Check sheet for the drawn part. Datum: minimum x, y, z corner. Units: mm. Round coordinates to 2 decimals unless told otherwise and drop trailing zeros. Write each loop counter-clockwise with the first axis right and the second up, starting at its lowest first coordinate (ties: lowest second). Pieces come first, ordered by that corner, then holes. Notation, with made-up numbers: (73, 25.5) - (124, 25.5) arc R22 ccw to (124, 52.5) - close; hole circle Ø11 at (-23, 5.5). An arc over 180 degrees is marked (long way). Answer as a JSON object with one key per item and string values. Group by question number.
Item 1: Gauge pin test, flat ends, axial feed: P1, Ø0.9, axis at y = 52, z = 2, coming from the +X side; P2, Ø1, axis at x = 209, z = 1, coming from the -Y side; P3, Ø1.5, axis at x = 117, z = 1, coming from the +Y side. Record the tip position at first contact, or that the pin passes through.
Item 2: Sectioned sample at B-B on x = 108.5. Record the boundary of the cut face in (y, z), plus the area to 3 significant figures.
Item 3: Sectioned sample at C-C on y = 51.5. Record the boundary of the cut face in (x, z), plus the area to 3 significant figures.
Item 4: Thickness scan on line 1 (Y direction, x = 125.5, z = 0.7); line 2 (X direction, y = 57.5, z = 2.75). Record the ranges inside material, lowest first.
Item 5: Sectioned sample at A-A on z = 1.1. Record the boundary of the cut face in (x, y).
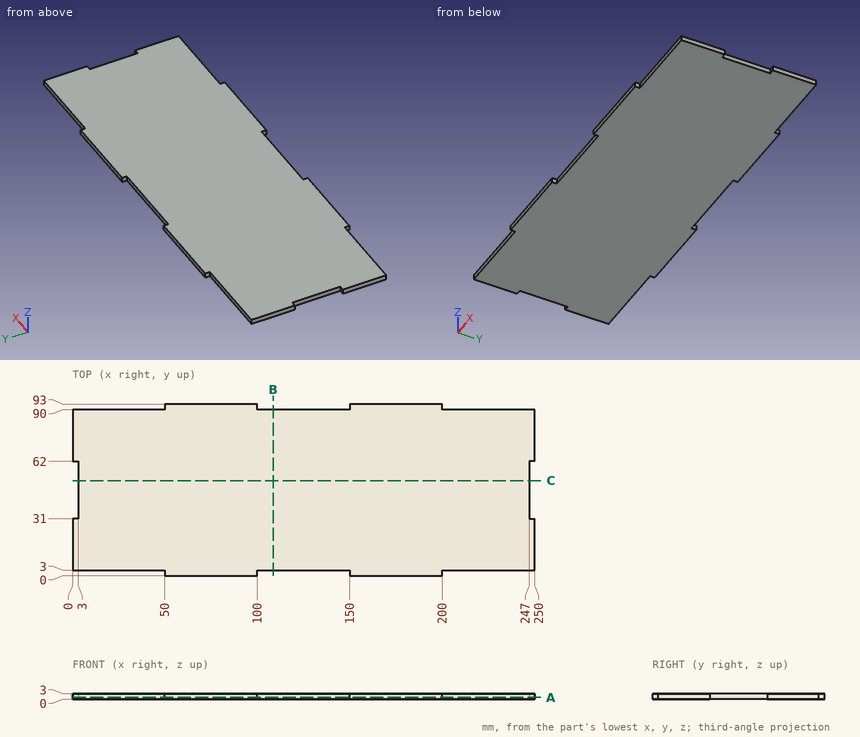
Completed:
{
 "1": {"P1": "x = 247", "P2": "y = 3", "P3": "y = 90"},
 "2": {"outline": "(3, 0) - (90, 0) - (90, 3) - (3, 3) - close", "area": "261 mm²"},
 "3": {"outline": "(3, 0) - (247, 0) - (247, 3) - (3, 3) - close", "area": "732 mm²"},
 "4": {"line 1": "3 to 90", "line 2": "3 to 247"},
 "5": {"outline": "(0, 3) - (50, 3) - (50, 0) - (100, 0) - (100, 3) - (150, 3) - (150, 0) - (200, 0) - (200, 3) - (250, 3) - (250, 31) - (247, 31) - (247, 62) - (250, 62) - (250, 90) - (200, 90) - (200, 93) - (150, 93) - (150, 90) - (100, 90) - (100, 93) - (50, 93) - (50, 90) - (0, 90) - (0, 62) - (3, 62) - (3, 31) - (0, 31) - close"}
}
